```python
from build123d import *

# Parameters (mm, degrees)
F1_DEPTH      = 24
F2_R          = 13
F3_R          = 5
F4_R          = 5
F4_R_2        = 2.5
F5_DEPTH      = 44.4
F7_DEPTH      = 15.7
F7_DEPTH_BACK = 25


with BuildPart() as f1:
    # F0 (on Front) → F1 (new body, symmetric)
    with BuildSketch(Plane.XZ):
        with BuildLine():
            ThreePointArc((-15, 0), (0, 15), (15, 0))
            Line((15, 0), (51, 0))
            Line((51, 0), (51, 41))
            Line((51, 41), (40, 41))
            Line((40, 41), (40, 11))
            Line((40, 11), (27.9105714739, 11))
            ThreePointArc((27.9105714739, 11), (0, 30), (-27.9105714739, 11))
            Line((-27.9105714739, 11), (-56, 11))
            Line((-56, 11), (-56, 0))
            Line((-56, 0), (-15, 0))
        make_face()
    extrude(amount=F1_DEPTH, both=True)

    # F2
    f2_edges = [f1.edges().sort_by_distance(p)[0] for p in [
        (-56, -24, 5.5),
        (-56, 24, 5.5),
    ]]
    fillet(f2_edges, radius=F2_R)

    # F3
    f3_edges = [f1.edges().sort_by_distance(p)[0] for p in [
        (45.5, -24, 41),
        (45.5, 24, 41),
        (-27.910571, 0, 11),
        (27.910571, 0, 11),
    ]]
    fillet(f3_edges, radius=F3_R)

    # F4 (on face) → F5 (cut, symmetric)
    with BuildSketch(Plane.XY.offset(11)):
        with Locations((-43, 12)):
            Circle(F4_R)
        with Locations((-43, -12)):
            Circle(F4_R)
        Circle(F4_R_2)
    extrude(amount=F5_DEPTH, both=True, mode=Mode.SUBTRACT)

    # F6 (on face) → F7 (cut, two sides)
    with BuildSketch(Plane.YZ.offset(51)) as f7_sk:
        with BuildLine():
            Line((6.5, 41), (-6.5, 41))
            Line((-6.5, 41), (-6.5, 25))
            ThreePointArc((-6.5, 25), (0, 18.5), (6.5, 25))
            Line((6.5, 25), (6.5, 41))
        make_face()
    extrude(amount=-F7_DEPTH, mode=Mode.SUBTRACT)
    extrude(f7_sk.sketch, amount=F7_DEPTH_BACK, mode=Mode.SUBTRACT)


solid = f1.part
```
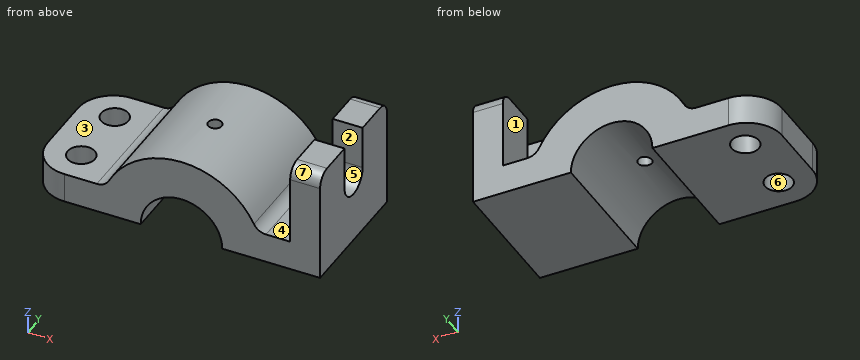
Input: part model. Units: mm. Frame: model coordinates. Face numbers are marked on the shaded views. A direction names the side the tool comes from. Round coordinates to 2 decimals unless told otherwise and drop trailing zeros. Write each loop counter-clockwise with the first axis right and the second up, starting at its lowest first coordinate (ties: lowest second). Pieces come first, ordered by that corner, then holes. Notation, with made-up numbers: (-39.75, 55.5) -> (-15.75, 55.5) arc R31 ccw to (-15.75, 88.5) -> close; hole circle Ø4 at (-12, -3). An arc over 180 degrees is marked (long way). Answer as CSV lines item,"result".
1. Section A-A (z = 5). Return the cut outline in (x, y).
Geometry says:
outline,"(-56, -11) arc R13 ccw to (-43, -24) -> (-14.14, -24) -> (-14.14, 24) -> (-43, 24) arc R13 ccw to (-56, 11) -> close; (14.14, -24) -> (51, -24) -> (51, 24) -> (14.14, 24) -> close; hole circle Ø10 at (-43, -12); hole circle Ø10 at (-43, 12)"
2. Reachability of the marked faces 1, 2 and 3 from +Z, -Z, +X, -X, +Y, -Y: full face, straight path, thin tool, end or side. Return the list, or none.
Geometry says:
face 1,"+Z, +Y, -Y"
face 2,"+Z, +X"
face 3,"+Z, -X, +Y, -Y"
3. Mould query, pull axis Y, two halves, no side actions, for the marked faces 4, 5, 6 and 7. Classes: +Y half, -Y half, draft (parallel to the pull), parting line (faces both ways), or undercut.
Geometry says:
face 4,"draft"
face 5,"undercut"
face 6,"undercut"
face 7,"-Y half"
4. Section B-B (y = 0). Return the cut outline in (x, z).
Geometry says:
outline,"(-56, 0) -> (-15, 0) arc R15 cw to (-2.5, 14.79) -> (-2.5, 29.9) arc R30 ccw to (-26.68, 13.71) arc R5 cw to (-31.13, 11) -> (-56, 11) -> close; (2.5, 14.79) arc R15 cw to (15, 0) -> (51, 0) -> (51, 18.5) -> (40, 18.5) -> (40, 11) -> (31.13, 11) arc R5 cw to (26.68, 13.71) arc R30 ccw to (2.5, 29.9) -> close"
5. Section C-C (x = -47). Return the cut outline in (y, z).
Geometry says:
outline,"(-23.37, 0) -> (-15, 0) -> (-15, 11) -> (-23.37, 11) -> close; (-9, 0) -> (9, 0) -> (9, 11) -> (-9, 11) -> close; (15, 0) -> (23.37, 0) -> (23.37, 11) -> (15, 11) -> close"
6. Contact query for flat-ended pins moving along their axis: P1, Ø8, axis at x = 32.5, y = -18, coming from the +Z side; P2, Ø4.5, axis at x = 0, y = 0, coming from the -Z side; P3, Ø10, axis at x = 34.5, y = -1, coming from the +Z side; P4, Ø4, axis at x = -3, y = -3, coming from the +Z side. Output: stop coordinate, or through.
Geometry says:
P1,"stops at z = 11.75"
P2,"passes through"
P3,"stops at z = 11.27"
P4,"stops at z = 29.98"
7. Section D-D (y = 13). Return the cut outline in (x, z), plus the area to 3 significant figures.
Geometry says:
outline,"(-55.85, 0) -> (-47.9, 0) -> (-47.9, 11) -> (-55.85, 11) -> close; (-38.1, 0) -> (-15, 0) arc R15 cw to (15, 0) -> (51, 0) -> (51, 41) -> (40, 41) -> (40, 11) -> (31.13, 11) arc R5 cw to (26.68, 13.71) arc R30 ccw to (-26.68, 13.71) arc R5 cw to (-31.13, 11) -> (-38.1, 11) -> close"
area,"1,820 mm^2"
8. Ray query, L1, parallel to Y at x = -43, z = 5.25; L2, parallel to Y at x = 0, z = 21.25; L3, parallel to X at y = -18.5, z = 11.5. Return the intervals inside material, ascending. Write a range as [from, to].
Geometry says:
L1,"y = [-24, -17], [-7, 7], [17, 24]"
L2,"y = [-24, -2.5], [2.5, 24]"
L3,"x = [-28.95, -9.63], [9.63, 28.95], [40, 51]"
